from build123d import *

# Parameters (mm, degrees)
SKETCH_1_W      = 30
SKETCH_1_H      = 20
EXTRUDE_1_DEPTH = 40
SKETCH_2_R      = 2
EXTRUDE_2_DEPTH = 5
SKETCH_3_RX     = 30
SKETCH_3_RY     = 5
EXTRUDE_3_DEPTH = 10
SKETCH_4_W      = 37.348500324
SKETCH_4_H      = 1
EXTRUDE_4_DEPTH = 2
EXTRUDE_START   = -2
EXTRUDE_5_DEPTH = 2


# Read off the part's stored shape, not the designer's step: 凸台-拉伸5
with BuildPart() as part:
    # 草图1 → 凸台-拉伸1 (new body)
    with BuildSketch(Plane.XY):
        with Locations((15, 10)):
            Rectangle(SKETCH_1_W, SKETCH_1_H)
    extrude(amount=EXTRUDE_1_DEPTH)

    # 草图2 → 凸台-拉伸2 (add)
    with BuildSketch(Plane.ZY):
        with Locations(Location((30, 10, 0), (0, 0, 180))):
            Circle(SKETCH_2_R)
    extrude(amount=EXTRUDE_2_DEPTH)

    # 草图3 → 凸台-拉伸3 (add)
    with BuildSketch(Plane.ZY.offset(5)):
        with Locations(Location((30, 10), (0, 0, -103.92099691))):
            Ellipse(SKETCH_3_RX, SKETCH_3_RY)
    extrude(amount=EXTRUDE_3_DEPTH)

    # 草图4 → 凸台-拉伸4 (add)
    with BuildSketch(Plane.ZY.offset(15)):
        with Locations((18.674250162, 39.574648358)):
            Rectangle(SKETCH_4_W, SKETCH_4_H)
    extrude(amount=-EXTRUDE_4_DEPTH)

    # 凸台-拉伸5 outline → 凸台-拉伸5 (add)
    with BuildSketch(Plane.ZY.offset(15).offset(EXTRUDE_START)):
        with BuildLine():
            Line((39.862468471, -21), (39.619125683, 32.967296936))
            add(Edge.make_bspline(
                [(39.619125683, 32.967296936), (39.589392589, 39.561347803), (37.614649654, 40.050686248)],
                knots=[5.629361553, 5.629361553, 5.629361553, 6.283185307, 6.283185307, 6.283185307], degree=2, weights=[1, 0.947038516, 1]))
            Line((37.614649654, 40.050686248), (37.348500324, 40.050855796))
            Line((37.348500324, 40.050855796), (37.348500324, 39.074648358))
            add(Edge.make_bspline(
                [(38.697434301, 33.514015855), (38.694345199, 38.494694197), (37.348500324, 39.074648358)],
                knots=[5.657287765, 5.657287765, 5.657287765, 6.250122592, 6.250122592, 6.250122592], degree=2, weights=[0.790463711, 0.847402464, 0.984462923]))
            Line((38.697434301, 33.514015855), (38.765118588, -21))
            Line((38.765118588, -21), (39.862468471, -21))
        make_face()
    extrude(amount=EXTRUDE_5_DEPTH)


solid = part.part
Source: CAD feature listing. Evaluate the final solid. Frame: model axes, mm. A direction names the side the tool comes from. Give positions to 0.01 mm unless a question says otherwise; leave off trailing zeros. Loops run counter-clockwise (first coordinate to the right, second up) from the corner with the lowest first, then second, coordinate; pieces in that order, holes last. Notation, with made-up numbers: (-3, -37) -> (11, -37) arc R24 cw to (11, -26) -> close; hole circle Ø9 at (-12, 28). An arc over 180 degrees is marked (long way). Use a Markdown table: item, result. Add a question column.
1) Section query C-C, the plane z = 22. Count the separate pieces of the cut face and the enclosed holes in it, then the cut area to 3 significant figures.
2) Section query B-B, the plane x = 25.5. Return the cut outline in (y, z).
3) Reachability of faces 1 (the face through (15, 10, 40)), 2 (the face through (15, 20, 20)) from +Z, -Z, +X, -X, +Y, -Y: full face, straight path, thin tool, end or side. Return the list, or none.
4) Section query A-A, the plane z = 7. Return the cut outline in (x, y).
5) Pull-direction query (Y, two-part tool) for faces 3 (the face through (-2.465, 9.399, 28.092)), 4 (the face through (0, 10, 20)), 5 (the face through (-14, 39.075, 18)), 6 (the face through (15, 0, 20)); classes: +Y half, -Y half, draft (parallel to the pull), parting line (faces both ways), or undercut.
6) First-contact query: pin 1 (2 mm diameter, centred on y = -12, z = 21.5, fed in from +X); pin 2 (1 mm diameter, centred on y = 12, z = 36, fed in from -X); pin 3 (22 mm diameter, centred on y = 9.5, z = 13, fed in from -X); pin 4 (12 mm diameter, centred on x = 17.5, z = 31.5, fed in from +Y). Flat tips, straight axial feed; report the tip coordinate or a pass-through.
7) Line query: line 1 along X through (y, z) = (17, 32.5); line 2 along X through (y, z) = (13, 21.5); line 3 along Y through (x, z) = (11.5, 38). Output: solid intervals per line, ascending. Write a range as [from, to].
Numbers:
| question | item | result |
|---|---|---|
| 1 | separate pieces | 3 |
| 1 | enclosed holes | 0 |
| 1 | area | 737 mm2 |
| 2 | outline | (0, 0) -> (20, 0) -> (20, 40) -> (0, 40) -> close |
| 3 | face 1 | +Z, +X, -X, +Y, -Y |
| 3 | face 2 | +Z, -Z, +X, +Y |
| 4 | outline | (-15, 39.07) -> (-13, 39.07) -> (-13, 40.07) -> (-15, 40.07) -> close; (0, 0) -> (30, 0) -> (30, 20) -> (0, 20) -> close |
| 5 | face 3 | parting line |
| 5 | face 4 | draft |
| 5 | face 5 | undercut |
| 5 | face 6 | -Y half |
| 6 | pin 1 | stops at x = -5 |
| 6 | pin 2 | stops at x = -15 |
| 6 | pin 3 | stops at x = 0 |
| 6 | pin 4 | stops at y = 20 |
| 7 | line 1 | x = [-15, -5], [0, 30] |
| 7 | line 2 | x = [0, 30] |
| 7 | line 3 | y = [0, 20] |
